Source: CAD feature listing. Evaluate the final solid. Frame: model axes, mm. A direction names the side the tool comes from. Round coordinates to 2 decimals unless told otherwise and drop trailing zeros. Write each loop counter-clockwise with the first axis right and the second up, starting at its lowest first coordinate (ties: lowest second). Pieces come first, ordered by that corner, then holes. Notation, with made-up numbers: (7.25, -39) -> (44.25, -39) arc R17 cw to (44.25, -17) -> close; hole circle Ø1 at (28, 48). An arc over 180 degrees is marked (long way). Put each result on its own line as item: value.
```python
from build123d import *

# Parameters (mm, degrees)
EXTRUDE_1_DEPTH = 14
EXTRUDE_2_DEPTH = 2.3
SKETCH_4_R      = 2.75
EXTRUDE_3_DEPTH = 3.5
SKETCH_5_R      = 1.7
EXTRUDE_4_DEPTH = 6.6


with BuildPart() as part:
    # Эскиз1 → Бобышка-Вытянуть1 (new body)
    with BuildSketch(Plane(origin=(0, 0, 0), x_dir=(0, 0, -1), z_dir=(1, 0, 0))):
        with BuildLine():
            Line((-3.35, -2.3), (-3.35, 2.3))
            ThreePointArc((-3.35, 2.3), (0, 5.65), (3.35, 2.3))
            Line((3.35, 2.3), (3.35, -2.3))
            ThreePointArc((3.35, -2.3), (0, -5.65), (-3.35, -2.3))
        make_face()
    extrude(amount=-EXTRUDE_1_DEPTH)

    # Эскиз3 → Бобышка-Вытянуть2 (add)
    with BuildSketch(Plane.ZY.offset(14)):
        with BuildLine():
            Line((2.75, 2.3), (2.75, -2.3))
            ThreePointArc((2.75, -2.3), (0, -5.05), (-2.75, -2.3))
            Line((-2.75, -2.3), (-2.75, 2.3))
            ThreePointArc((-2.75, 2.3), (0, 5.05), (2.75, 2.3))
        make_face()
    extrude(amount=EXTRUDE_2_DEPTH)

    # Эскиз4 → Бобышка-Вытянуть3 (add)
    with BuildSketch(Plane.ZY.offset(16.3)):
        Circle(SKETCH_4_R)
    extrude(amount=EXTRUDE_3_DEPTH)

    # По траектории1: sweep along a path in Эскиз6
    with BuildLine(Plane.XY) as sweep_1_path:
        Line((-19.8, 0), (-24.776161806, 0))
        ThreePointArc((-24.776161806, 0), (-30.870449905, -0.986593903), (-36.342181829, -3.845591055))
    # Эскиз5 → По траектории1 (sweep)
    with BuildSketch(Plane.ZY.offset(19.8)):
        Circle(SKETCH_5_R)
    sweep(path=sweep_1_path.line)

    # Эскиз7 → Бобышка-Вытянуть4 (add)
    with BuildSketch(Plane(origin=(0, 0, 0), x_dir=(0, 0, -1), z_dir=(1, 0, 0))):
        with BuildLine():
            Line((-1.2, -2.925), (-1.2, 2.925))
            ThreePointArc((-1.2, 2.925), (0, 4.125), (1.2, 2.925))
            Line((1.2, 2.925), (1.2, -2.925))
            ThreePointArc((1.2, -2.925), (0, -4.125), (-1.2, -2.925))
        make_face()
        with BuildLine():
            Line((-0.55, -3.15), (-0.55, 3.15))
            ThreePointArc((-0.55, 3.15), (0, 3.7), (0.55, 3.15))
            Line((0.55, 3.15), (0.55, -3.15))
            ThreePointArc((0.55, -3.15), (0, -3.7), (-0.55, -3.15))
        make_face(mode=Mode.SUBTRACT)
    extrude(amount=EXTRUDE_4_DEPTH)


solid = part.part
```
Q1. Cut plane C-C on x = -10. Output: boundary loops of the cut face in (y, z).
Ans:
outline: (-2.3, -3.35) -> (2.3, -3.35) arc R3.35 ccw to (2.3, 3.35) -> (-2.3, 3.35) arc R3.35 ccw to start
Q2. Cut plane B-B on z = 0. Output: boundary loops of the cut face in (x, y) (3 decimals), and give its area (3 significant figures).
Ans:
outline: (-37.36, -2.484) -> (-35.324, -5.207) arc R17.616 cw to (-24.776, -1.7) -> (-19.8, -1.7) -> (-19.8, -2.75) -> (-16.3, -2.75) -> (-16.3, -5.05) -> (-14, -5.05) -> (-14, -5.65) -> (0, -5.65) -> (0, -4.125) -> (6.6, -4.125) -> (6.6, -3.7) -> (0, -3.7) -> (0, 3.7) -> (6.6, 3.7) -> (6.6, 4.125) -> (0, 4.125) -> (0, 5.65) -> (-14, 5.65) -> (-14, 5.05) -> (-16.3, 5.05) -> (-16.3, 2.75) -> (-19.8, 2.75) -> (-19.8, 1.7) -> (-24.776, 1.7) arc R21.016 ccw to start
area: 265 mm^2
Q3. Reachability of faces 4 (the cylindrical face through (3.3, 3.7, 0)), 5 (the flat face through (-19.8, 0, 2)), 6 (the cylindrical face through (-15.13, -5.05, 0.06)), 7 (the cylindrical face through (3.254, -4.125, -0.026)), 8 (the flat face through (-15, 0, 2.75)) from +Z, -Z, +X, -X, +Y, -Y: full face, straight path, thin tool, end or side. Return the list, or none.
Ans:
face 4: +X
face 5: none
face 6: -Y
face 7: +X, -Y
face 8: +Z, -X, +Y, -Y
Q4. Material intervals for line 1 (X direction, y = -2, z = -2); line 2 (X direction, y = 1, z = 3.25); line 3 (Z direction, x = 3.5, y = -3.25), sorted ascending. Write a range as [from, to].
Ans:
line 1: x = [-16.3, 0]
line 2: x = [-14, 0]
line 3: z = [-1.16, -0.54], [0.54, 1.16]
Q5. Cut plane A-A on x = 2. Output: boundary loops of the cut face in (y, z) (3 decimals).
Ans:
outline: (-2.925, -1.2) -> (2.925, -1.2) arc R1.2 ccw to (2.925, 1.2) -> (-2.925, 1.2) arc R1.2 ccw to start; hole (-3.15, -0.55) -> (3.15, -0.55) arc R0.55 ccw to (3.15, 0.55) -> (-3.15, 0.55) arc R0.55 ccw to start
Q6. Draft query along Y for faces 1 (the flat face through (3, 0, 0.55)), 2 (the flat face through (-16.3, 3, 0)), 3 (the flat face through (-36.356, -3.827, 0.024)). Return one class per face: +Y half, -Y half, draft (parallel to the pull), parting line (faces both ways), or undercut.
Ans:
face 1: undercut
face 2: draft
face 3: -Y half
Q7. Pin query (flat end, axial travel): pin 1 (1.9 mm diameter, centred on x = 2.5, y = 1, fed in from +Z); pin 2 (1.5 mm diameter, centred on x = -25.5, z = 1, fed in from -Y); pin 3 (4.5 mm diameter, centred on x = 3, y = -1, fed in from -Z). Return the tip coordinate at first contact, or that it passes through.
Ans:
pin 1: stops at z = 1.2
pin 2: stops at y = -1.7
pin 3: stops at z = -1.2
